from build123d import *

# Parameters (mm, degrees)
F0_R     = 4.5
F1_DEPTH = 8
F0_R_2   = 29
F0_R_3   = 27
F2_DEPTH = 4


with BuildPart() as f1:
    # F0 (on Front) → F1 (new body)
    with BuildSketch(Plane.XZ):
        Circle(F0_R)
    extrude(amount=F1_DEPTH)

    # F0 (on Front) → F2 (join)
    with BuildSketch(Plane.XZ):
        Circle(F0_R_2)
        Circle(F0_R_3, mode=Mode.SUBTRACT)
        Circle(F0_R_3)
        with BuildLine():
            Line((-25.3947422835, -5), (-5, -5))
            Line((-5, -5), (-5, -25.3947395831))
            ThreePointArc((-5, -25.3947395831), (-18.3578630178, -18.3578620861), (-25.3947422835, -5))
        make_face(mode=Mode.SUBTRACT)
        with BuildLine():
            ThreePointArc((4.5, -21.5), (0, -26), (-4.5, -21.5))
            Line((-4.5, -21.5), (-2.25, -7.75))
            ThreePointArc((-2.25, -7.75), (0, -5.5), (2.25, -7.75))
            Line((2.25, -7.75), (4.5, -21.5))
        make_face(mode=Mode.SUBTRACT)
        with BuildLine():
            Line((5, -25.3947395831), (5, -5))
            Line((5, -5), (25.3947422835, -5))
            ThreePointArc((25.3947422835, -5), (18.3578630178, -18.3578620861), (5, -25.3947395831))
        make_face(mode=Mode.SUBTRACT)
        with BuildLine():
            ThreePointArc((-20.0656793303, -4.2652929813), (-25.940935623, -0.7266985565), (-21.5, 4.5))
            Line((-21.5, 4.5), (-7.75, 2.25))
            ThreePointArc((-7.75, 2.25), (-5.5, 0), (-7.75, -2.25))
            Line((-7.75, -2.25), (-20.0656793303, -4.2652929813))
        make_face(mode=Mode.SUBTRACT)
        with BuildLine():
            Line((-5, 25.3947422835), (-5, 5))
            Line((-5, 5), (-25.3947422835, 5))
            ThreePointArc((-25.3947422835, 5), (-18.35786369, 18.35786369), (-5, 25.3947422835))
        make_face(mode=Mode.SUBTRACT)
        Circle(F0_R, mode=Mode.SUBTRACT)
        with BuildLine():
            ThreePointArc((7.75, -2.25), (5.5, 0), (7.75, 2.25))
            Line((7.75, 2.25), (21.4941852602, 4.5))
            ThreePointArc((21.4941852602, 4.5), (25.9941852602, 0), (21.4941852602, -4.5))
            Line((21.4941852602, -4.5), (7.75, -2.25))
        make_face(mode=Mode.SUBTRACT)
        with BuildLine():
            ThreePointArc((-4.5, 21.5), (0, 26), (4.5, 21.5))
            Line((4.5, 21.5), (2.25, 7.75))
            ThreePointArc((2.25, 7.75), (0, 5.5), (-2.25, 7.75))
            Line((-2.25, 7.75), (-4.5, 21.5))
        make_face(mode=Mode.SUBTRACT)
        with BuildLine():
            Line((25.3947422835, 5), (5, 5))
            Line((5, 5), (5, 25.3947422835))
            ThreePointArc((5, 25.3947422835), (18.35786369, 18.35786369), (25.3947422835, 5))
        make_face(mode=Mode.SUBTRACT)
    extrude(amount=F2_DEPTH)


solid = f1.part
Read the model definition and answer for the solid it produces. Units are mm, in the model's axes. A direction names the side the tool comes from. Round coordinates to 2 decimals unless told otherwise and drop trailing zeros. Loops run counter-clockwise (first coordinate to the right, second up) from the corner with the lowest first, then second, coordinate; pieces in that order, holes last.
Q1. Section B-B on y = -3.25 is taken. Give the number of separate pieces and of enclosed holes in the cut face, and give its area (3 significant figures).
Q2. Consider probe 1 along Z at (x, y) = (-21.5, -3); probe 2 along X at (y, z) = (-0.75, 18.5); probe 3 along Z at (x, y) = (12.5, -0.5). Determine where each line is inside the solid, lowest interval first.
Q3. Section C-C on z = -13.5 is taken. Write down the section's boundary in (x, y), and give its area (3 significant figures).
Q4. Which of the six approach directions +Z, -Z, +X, -X, +Y, -Y give full straight-line access (tool end or side, diameter ignored) to faces 1 (the face through (4.2, -4, 2.3)), 2 (the face through (0, -2, 26))?
Q5. Section A-A on x = 0 is taken. Write down the section's boundary in (y, z).
Q6. Each of these flat-tipped pins is pushed along its axis until it touches: pin 1 (2 mm diameter, centred on x = 18, y = -2.5, fed in from -Z); pin 2 (4 mm diameter, centred on x = -5.5, z = 2.5, fed in from +Y); pin 3 (1.2 mm diameter, centred on x = 19.5, y = -2.5, fed in from +Z); pin 4 (1.2 mm diameter, centred on x = -18.5, y = -1.5, fed in from -Z). Where does it stop, or does it pass through?
Q7. Determine the mould class of faces 3 (the face through (0, 0, 2)), 4 (the face through (3.39, -1.97, 14.72)), 5 (the face through (13.38, -1.97, -25.73)) for opening direction X: released by +X, released by -X, zero draft, split by the parting line, or undercut.
Q8. Section D-D on x = 6.5 is taken. Write down the section's boundary in (y, z).
Output:
1. separate pieces: 1
1. enclosed holes: 8
1. area: 930 mm2
2. probe 1: z = -19.46 to -14.54, -5 to -4.5, 4.5 to 5, 14.54 to 19.46
2. probe 2: x = -22.33 to -18.21, -5 to -4.01, 4.01 to 5, 18.21 to 22.33
2. probe 3: z = -26.17 to -22.73, -5 to -3.03, 3.03 to 5, 22.73 to 26.17
3. outline: (-25.67, -4) - (-22.16, -4) - (-22.16, 0) - (-25.67, 0) - close; (-5, -4) - (-3.19, -4) - (-3.19, 0) - (-5, 0) - close; (3.19, -4) - (5, -4) - (5, 0) - (3.19, 0) - close; (22.16, -4) - (25.67, -4) - (25.67, 0) - (22.16, 0) - close
3. area: 42.5 mm2
4. face 1: -Y
4. face 2: +Y, -Y
5. outline: (-8, -4.5) - (-4, -4.5) - (-4, -5.5) - (0, -5.5) - (0, 5.5) - (-4, 5.5) - (-4, 4.5) - (-8, 4.5) - close; (-4, -29) - (0, -29) - (0, -26) - (-4, -26) - close; (-4, 26) - (0, 26) - (0, 29) - (-4, 29) - close
6. pin 1: stops at z = -23.49
6. pin 2: stops at y = 0
6. pin 3: stops at z = 22
6. pin 4: stops at z = -22.82
7. face 3: zero draft
7. face 4: undercut
7. face 5: split by the parting line
8. outline: (-4, -28.26) - (0, -28.26) - (0, -25.07) - (-4, -25.07) - close; (-4, -5) - (0, -5) - (0, -1.87) - (-4, -1.87) - close; (-4, 1.87) - (0, 1.87) - (0, 5) - (-4, 5) - close; (-4, 25.07) - (0, 25.07) - (0, 28.26) - (-4, 28.26) - close
